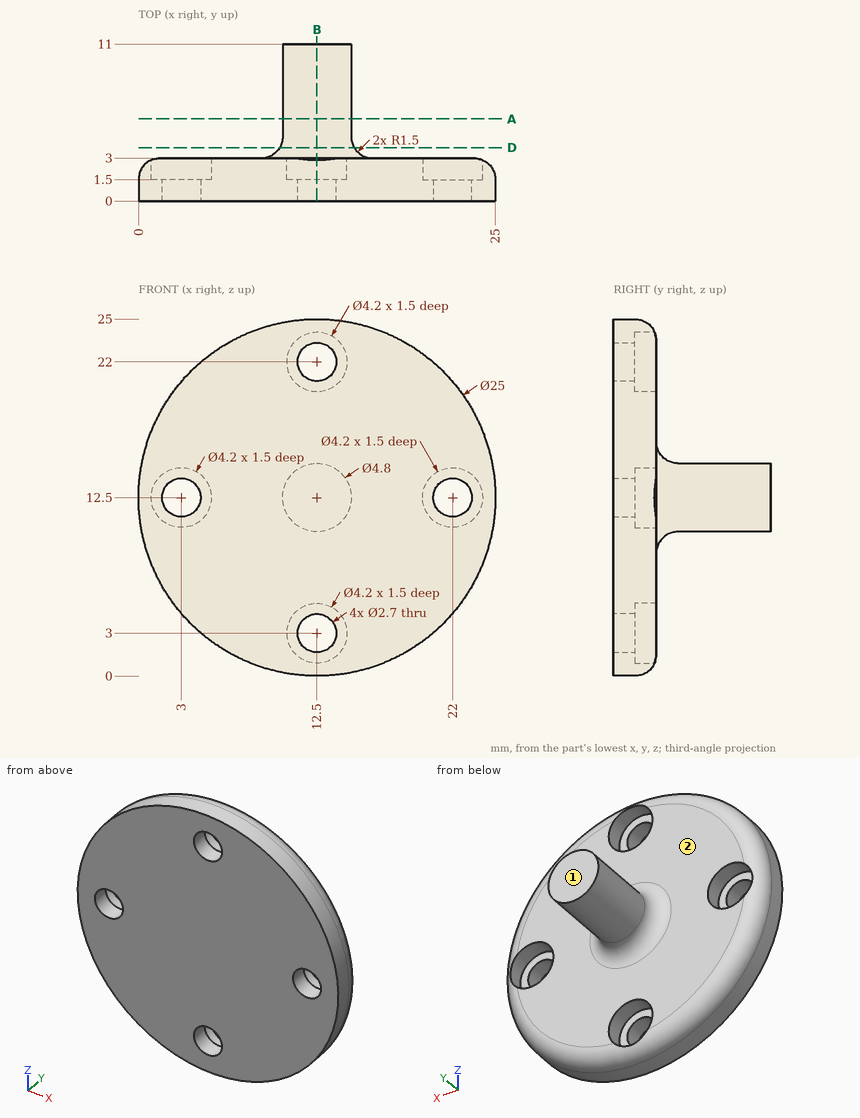
Source: three-view drawing plus pictorial views. Frame: mm from the lowest corner of the part. A direction names the side the tool comes from. Give positions to 0.01 mm unless a question says otherwise; leave off trailing zeros. Order: outer loops, then holes, each group sorted by start corner. A loop starts at its lowest first (then second) coordinate and runs counter-clockwise, first axis right, second up. Notation, with made-up numbers: M 83,40 L 131,40 A20 cw 131,76 Z; hole C -39.75,70 d6. An arc over 180 degrees is marked long. One line per question, with ' | ' between items. Start each with the question number.
1. Section query D-D (y = 3.75). Return the cut outline in (x, z).
2. Section query B-B (x = 12.5). Count the separate pieces of the cut face and the enclosed holes in it, and give its area (3 significant figures).
3. Section query A-A (y = 5.75). Return the cut outline in (x, z), and give its area (3 significant figures).
4. Material intervals for probe 1 along Y at (x, z) = (11.75, 1.5); probe 2 along Y at (x, z) = (19, 20); probe 3 along X at (y, z) = (2.5, 3), sorted ascending. Write a range as [from, to].
5. Access query for the marked faces 1 and 2. Directions: +Z, -Z, +X, -X, +Y, -Y. A direction counts if a zero-diameter tool reaches every point of the face in a straight line with its end or side. Return the directions, or none.
6. First-contact query: pin 1 Ø5 at (y, z) = (10, 19) entering from +X; pin 2 Ø12 at (x, z) = (6.5, 12.5) entering from -Y; pin 3 Ø3.5 at (x, z) = (12.5, 2) entering from +Y; pin 4 Ø3.5 at (x, z) = (3, 12.5) entering from +Y. Flat tips, straight axial feed; report the tip coordinate or a pass-through.
Here are the results:
1) outline: C 12.5,12.5 d5.2
2) separate pieces: 3 | enclosed holes: 0 | area: 92.7 mm²
3) outline: C 12.5,12.5 d4.8 | area: 18.1 mm²
4) probe 1: [0, 1.5] | probe 2: [0, 3] | probe 3: [4.98, 10.4], [14.6, 20.02]
5) face 1: +Z, -Z, +X, -X, +Y | face 2: +Y
6) pin 1: through | pin 2: y = 0 | pin 3: y = 3 | pin 4: y = 1.5
